Autodesk Inventor part; units mm, degrees
ref_plane "YZ Plane" through (0, 0, 0) normal (1, 0, 0) x (0, 1, 0)
ref_plane "XZ Plane" through (0, 0, 0) normal (0, 1, 0) x (-1, 0, 0)
ref_plane "XY Plane" through (0, 0, 0) normal (0, 0, 1) x (1, 0, 0)
sketch "Sketch1" plane through (0, 0, 0) normal (0, 0, 1) x (1, 0, 0)
  line L0 (-12.1708, 16.0073) -> (13.2292, 16.0073)
  line L1 (13.2292, 16.0073) -> (13.2292, -34.7927)
  line L2 (13.2292, -34.7927) -> (-12.1708, -34.7927)
  line L3 (-12.1708, -34.7927) -> (-12.1708, 16.0073)
  line L4 (11.9592, 14.7373) -> (-10.9008, 14.7373)
  line L5 (-10.9008, 14.7373) -> (-10.9008, -33.5227)
  line L6 (-10.9008, -33.5227) -> (11.9592, -33.5227)
  line L7 (11.9592, -33.5227) -> (11.9592, 14.7373)
  point P0 (0, 0)
  dimension "d0" = 25.4
  dimension "d1" = 50.8
  dimension "d2" = 1.27
extrude "Extrusion1" add sketch "Sketch1" along normal blind 558.8
sketch "Sketch2" plane through (-12.1708, 16.0073, 0) normal (0, 1, 0) x (1, 0, 0)
  circle A0 centre (12.7, -12.7) radius 1.7272
  line L0 (25.4, 0) -> (0, 0)
  line L1 (0, 0) -> (0, -558.8)
  point P0 (12.1708, 0)
  dimension "d5" = 3.4544
  dimension "d6" = 12.7
  dimension "d7" = 12.7
extrude "Extrusion2" cut sketch "Sketch2" against normal through all
pattern_linear "Rectangular Pattern1" count 56 spacing 25.4 along (0, 0, 1) of "Extrusion2"
sketch "Sketch3" plane through (0, 0, 558.8) normal (0, 0, 1) x (1, 0, 0)
  line L0 (-12.1708, 16.0073) -> (-12.1708, -34.7927)
  line L1 (-12.1708, -34.7927) -> (13.2292, -34.7927)
  line L2 (-12.1708, 16.0073) -> (0.5292, 16.0073)
  line L3 (0.5292, 16.0073) -> (0.5292, -34.7927)
  line L4 (0.5292, -34.7927) -> (-12.1708, -34.7927)
  line L5 (-12.1708, -34.7927) -> (-12.1708, 16.0073)
  line L6 (11.9592, -33.5227) -> (-10.9008, -33.5227)
  line L7 (-10.9008, -33.5227) -> (-10.9008, 14.7373)
  line L8 (0.5292, -33.5227) -> (-10.9008, -33.5227)
  line L9 (-10.9008, -33.5227) -> (-10.9008, 14.7373)
  line L10 (-10.9008, 14.7373) -> (0.5292, 14.7373)
  line L11 (0.5292, 14.7373) -> (0.5292, -33.5227)
  point P0 (0, 0)
  point P1 (0.5292, -33.5227)
  dimension "d15" = 12.7
extrude "Extrusion3" cut sketch "Sketch3" against normal blind 558.8 contours L2 L3 L10 L7 L6 L1 L0
sketch "Sketch4" plane through (13.2292, -34.7927, 0) normal (1, 0, 0) x (0, 0, -1)
  line L0 (-558.8, 0) -> (-558.8, 50.8)
  line L1 (-558.8, 25.4) -> (0, 25.4) construction
  line L2 (0, 0) -> (0, 50.8)
  circle A0 centre (-533.4, 25.4) radius 9.525
  circle A1 centre (-469.9, 25.4) radius 9.525
  circle A2 centre (-495.3, 25.4) radius 2.5781
  circle A3 centre (-444.5, 25.4) radius 2.5781
  circle A4 centre (-469.9, 25.4) radius 25.4 construction
  circle A5 centre (-25.4, 25.4) radius 14.2875
  line L3 (-554.0222, 13.4938) -> (-512.7778, 13.4938) construction
  line L4 (-512.7778, 13.4938) -> (-512.7778, 37.3062) construction
  line L5 (-512.7778, 37.3062) -> (-554.0222, 37.3062) construction
  line L6 (-554.0222, 37.3062) -> (-554.0222, 13.4938) construction
  line L7 (-554.0222, 13.4938) -> (-512.7778, 37.3062) construction
  line L8 (-512.7778, 13.4938) -> (-554.0222, 37.3062) construction
  point P0 (0, 34.7927)
  dimension "d18" = 28.575
  dimension "d19" = 50.8
  dimension "d20" = 5.1562
  dimension "d21" = 19.05
  dimension "d22" = 25.4
  dimension "d23" = 25.4
  dimension "d24" = 19.05
  dimension "d25" = 63.5
  dimension "d26" = 47.625
  dimension "d27" = 60
extrude "Extrusion4" cut sketch "Sketch4" against normal through all
sketch "Sketch5" plane through (13.2292, -34.7927, 0) normal (1, 0, 0) x (0, 0, -1)
  circle A0 centre (-533.4, 25.4) radius 9.525
  circle A1 centre (-533.4, 25.4) radius 23.8125 construction
  line L0 (-554.0222, 37.3063) -> (-512.7778, 13.4937) construction
  line L1 (-554.0222, 13.4938) -> (-512.7778, 37.3062) construction
  line L2 (0, 0) -> (-558.8, 0)
  circle A2 centre (-554.0222, 37.3063) radius 2.1463
  circle A3 centre (-512.7778, 37.3062) radius 2.1463
  circle A4 centre (-512.7778, 13.4937) radius 2.1463
  circle A5 centre (-554.0222, 13.4938) radius 2.1463
  point P0 (0, 34.7927)
  dimension "d30" = 47.625
  dimension "d31" = 60
  dimension "d32" = 30
  dimension "d33" = 4.2926
extrude "Extrusion5" cut sketch "Sketch5" against normal through all contours A2 | A3 | A4 | A5
equation "\"d3\" = d13"
equation "\"d16\" = d13"
equation "\"d14\" = d13"
equation "\"d10\" = d14"
equation "\"d13\" = 558.8"
properties part number "VerseFrame 18in C Channel"
Could you check a few things on this model? Use its own coordinates, in mm. A direction names the side the tool comes from. Coordinates: 2 decimals unless noted, no trailing zeros. Order: outer loops, then holes, each group sorted by start corner. A loop starts at its lowest first (then second) coordinate and runs counter-clockwise, first axis right, second up. Notation, with made-up numbers: (52.5, 27.25) - (72.5, 27.25) arc R25 cw to (72.5, 41.25) - close; hole circle Ø4 at (1, 62.5). An arc over 180 degrees is marked (long way). Answer in a Markdown table with one row per item. Add a question column.
(1) If we section it at C-C, the plane z = 454: Please give me the cut outline in (x, y), then the cut area to 3 significant figures.
(2) If we mould it in two halves opening along Y, with no side actions, what happens to faces 3 (the face through (12.6, -23.34, 28.5)), 4 (the face through (7, -34.793, 275)), 5 (the face through (13, -9, 0)), 6 (the face through (12.603, -6.532, 524.315))? For each: released by +Y, released by -Y, zero draft, split by the parting line, or undercut.
(3) I need wall thicknesses on L1, parallel to Y at x = 9, z = 282; L2, parallel to Y at x = 12.45, z = 469.9; L3, parallel to X at y = 10, z = 109. Which ranges of each line are inside material? Lowest first, please.
(4) On a 3-axis mill with a long thin cutter (end or side, diameter ignored), from which of +Z, -Z, +X, -X, +Y, -Y can I reach the whole of each face in a straight line? I mean faces 1 (the face through (13, -9, 558.8)), 2 (the face through (6, 14.737, 275)). Say none if no direction works.
(5) If we section it at A-A, the plane x = 9.25: Please give me the cut outline in (y, z).
(6) If we section it at B-B, the plane z = 533.4: Please give me the cut outline in (x, y).
(7) Will these pins go through, and if not, where does the flat tip stop? pin 1 (2 mm diameter, centred on y = -7.5, z = 77.5, fed in from -X); pin 2 (11.5 mm diameter, centred on y = -9.39, z = 533.4, fed in from -X).
Results are:
| question | item | result |
|---|---|---|
| 1 | outline | (0.53, -34.79) - (13.23, -34.79) - (13.23, 16.01) - (0.53, 16.01) - (0.53, 14.74) - (11.96, 14.74) - (11.96, -33.52) - (0.53, -33.52) - close |
| 1 | area | 93.5 mm2 |
| 2 | face 3 | undercut |
| 2 | face 4 | released by -Y |
| 2 | face 5 | zero draft |
| 2 | face 6 | undercut |
| 3 | L1 | y = -34.79 to -33.52, 14.74 to 16.01 |
| 3 | L2 | y = -34.79 to -18.92, 0.13 to 16.01 |
| 3 | L3 | x = 11.96 to 13.23 |
| 4 | face 1 | +Z, +X, -X, +Y, -Y |
| 4 | face 2 | +Z, -Z, -X |
| 5 | outline | (-34.79, 0) - (-33.52, 0) - (-33.52, 558.8) - (-34.79, 558.8) - close; (14.74, 0) - (16.01, 0) - (16.01, 558.8) - (14.74, 558.8) - close |
| 6 | outline | (0.53, -34.79) - (13.23, -34.79) - (13.23, -18.92) - (11.96, -18.92) - (11.96, -33.52) - (0.53, -33.52) - close; (0.53, 14.74) - (11.96, 14.74) - (11.96, 0.13) - (13.23, 0.13) - (13.23, 16.01) - (0.53, 16.01) - close |
| 7 | pin 1 | stops at x = 11.96 |
| 7 | pin 2 | passes through |
